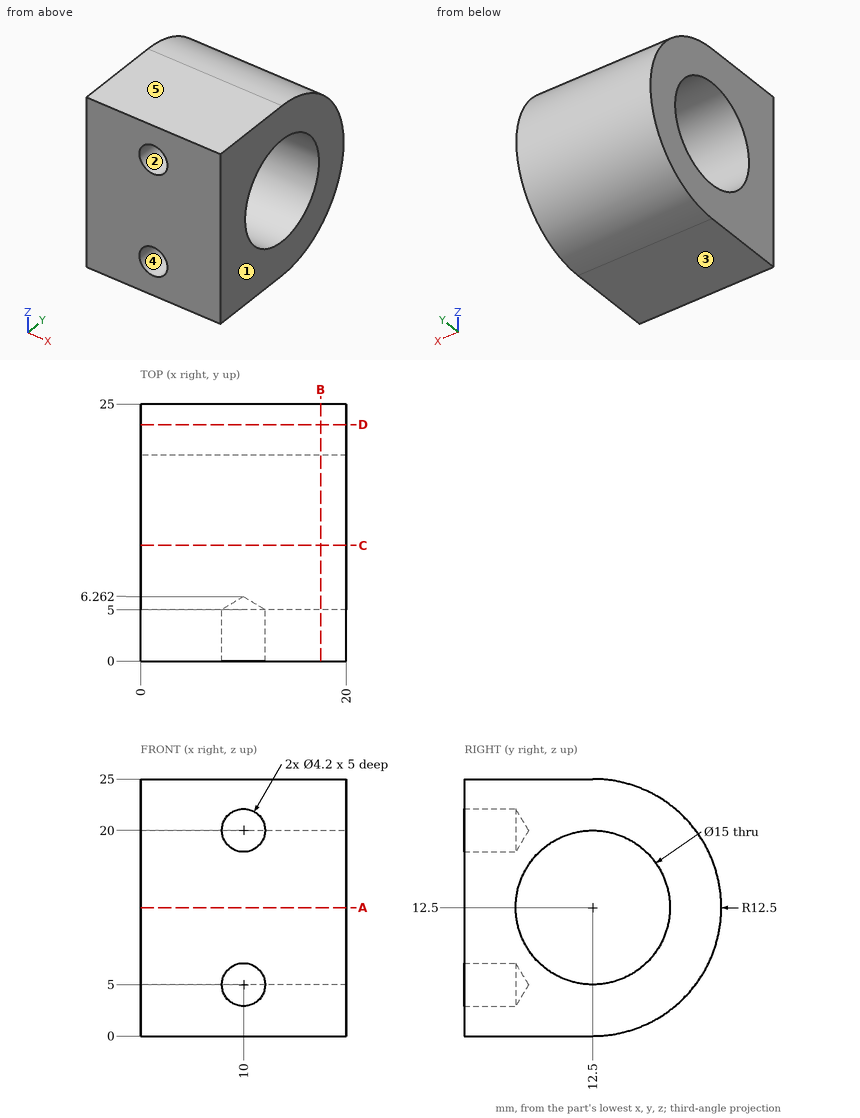
For this review, use the dimensioned drawing (mm, ordinates from the lowest corner) and the shaded views. A direction names the side the tool comes from. Give positions to 0.01 mm unless a question says otherwise; leave off trailing zeros. Loops run counter-clockwise (first coordinate to the right, second up) from the corner with the lowest first, then second, coordinate; pieces in that order, holes last. Notation, with made-up numbers: (39.25, 55.5) - (49.25, 55.5) arc R6 ccw to (49.25, 61.5) - close; hole circle Ø4 at (70.5, 18). An arc over 180 degrees is marked (long way). Write each question's results on one line, items separated by ' | '.
(1) For the marked faces 4 and 5, list the 3-axis set-ups (+Z, -Z, +X, -X, +Y, -Y) from which the entire face can be reached by the end or side of a thin tool; tool diameter is ignored.
Conclusion:
face 4: -Y | face 5: +Z, +X, -X, +Y, -Y
(2) Take a section at A-A (z = 12.5). Give the boundary of the cut face in (x, y).
Conclusion:
outline: (0, 0) - (20, 0) - (20, 5) - (0, 5) - close; (0, 20) - (20, 20) - (20, 25) - (0, 25) - close
(3) Take a section at C-C (y = 11.25). Give the boundary of the cut face in (x, z) (3 decimals), then the cut area to 3 significant figures.
Conclusion:
outline: (0, 0) - (20, 0) - (20, 5.105) - (0, 5.105) - close; (0, 19.895) - (20, 19.895) - (20, 25) - (0, 25) - close | area: 204 mm^2
(4) Take a section at B-B (x = 17.5). Give the boundary of the cut face in (y, z), then the cut area to 3 significant figures.
Conclusion:
outline: (0, 0) - (12.5, 0) arc R12.5 ccw to (12.5, 25) - (0, 25) - close; hole circle Ø15 at (12.5, 12.5) | area: 381 mm^2
(5) For line 1 along Z through (x, y) = (10, 2); line 2 along X through (y, z) = (1.9, 5); line 3 along Y through (x, z) = (7.25, 12.5), list the stretches that pass through material, from the lowest coordinate up.
Conclusion:
line 1: 0 to 2.9, 7.1 to 17.9, 22.1 to 25 | line 2: 0 to 7.9, 12.1 to 20 | line 3: 0 to 5, 20 to 25
(6) Take a section at D-D (y = 23). Give the boundary of the cut face in (x, z), then the cut area to 3 significant figures.
Conclusion:
outline: (0, 5.72) - (20, 5.72) - (20, 19.28) - (0, 19.28) - close | area: 271 mm^2
(7) For pin 1 Ø10 at (x, z) = (8.5, 20) entering from +Y; pin 2 Ø4 at (y, z) = (22, 7) entering from -X; pin 3 Ø1.5 at (x, z) = (9, 8) entering from +Y; pin 4 Ø2.5 at (x, z) = (10, 5) entering from -Y, all flat-tipped, find the tip position at first contact; note any pin that passes through.
Conclusion:
pin 1: y = 24.75 | pin 2: x = 0 | pin 3: y = 24.42 | pin 4: y = 5.51
(8) Draft analysis for pull direction Z (two halves, no side actions). For the marked faces 1, 2 and 3, state which applies: +Z half, -Z half, draft (parallel to the pull), parting line (faces both ways), or undercut.
Conclusion:
face 1: draft | face 2: undercut | face 3: -Z half
